Part model, mm, in its own coordinate system. Give positions to 0.01 mm unless a question says otherwise; leave off trailing zeros. Loops run counter-clockwise (first coordinate to the right, second up) from the corner with the lowest first, then second, coordinate; pieces in that order, holes last. Notation, with made-up numbers: (59, 36) -> (102, 36) arc R21 cw to (102, 43) -> close; hole circle Ø11 at (26.5, 1.25). An arc over 180 degrees is marked (long way). One line per question, with ' | ' between items.
```python
from build123d import *

# Parameters (mm, degrees)
SKETCH1_R           = 1.6
BOSS_EXTRUDE2_DEPTH = 5
BOSS_EXTRUDE3_DEPTH = 10
CHAMFER1_SIZE       = 1.5
FILLET1_R           = 10
FILLET2_R           = 1


with BuildPart() as part:
    # Sketch1 → Boss-Extrude2 (new body)
    with BuildSketch(Plane(origin=(0, 0, 0), x_dir=(0, 1, 0), z_dir=(0, 0, 1))):
        with BuildLine():
            Line((-82.0624762, -24), (82.0624762, -24))
            ThreePointArc((82.0624762, -24), (0, -85.5), (-82.0624762, -24))
        make_face()
        with Locations(Location((-20, -75, 0), (0, 0, 270))):
            Circle(SKETCH1_R, mode=Mode.SUBTRACT)
        with Locations(Location((20, -75, 0), (0, 0, 90))):
            Circle(SKETCH1_R, mode=Mode.SUBTRACT)
        with Locations(Location((-69.5, -28.2, 0), (0, 0, 270))):
            Circle(SKETCH1_R, mode=Mode.SUBTRACT)
        with Locations(Location((69.5, -28.2, 0), (0, 0, 90))):
            Circle(SKETCH1_R, mode=Mode.SUBTRACT)
    extrude(amount=BOSS_EXTRUDE2_DEPTH)

    # Sketch2 → Boss-Extrude3 (add)
    with BuildSketch(Plane.XY.offset(5)):
        with BuildLine():
            Line((60, 45), (24, 45))
            Line((24, 45), (24, 40))
            Line((24, 40), (63.442887702, 40))
            ThreePointArc((63.442887702, 40), (61.772053803, 42.534848876), (60, 45))
        make_face()
        with BuildLine():
            Line((24, -45), (24, -40))
            Line((24, -40), (63.442887702, -40))
            ThreePointArc((63.442887702, -40), (61.772053803, -42.534848876), (60, -45))
            Line((60, -45), (24, -45))
        make_face()
    extrude(amount=BOSS_EXTRUDE3_DEPTH)

    # Chamfer1
    chamfer1_edges = [part.edges().sort_by_distance(p)[0] for p in [
        (76.6, 20, 5),
        (26.6, -69.5, 5),
        (29.8, 69.5, 5),
        (73.4, -20, 5),
    ]]
    chamfer(chamfer1_edges, length=CHAMFER1_SIZE)

    # Fillet1
    fillet1_edges = [part.edges().sort_by_distance(p)[0] for p in [
        (42, -45, 5),
        (42, 45, 5),
    ]]
    fillet(fillet1_edges, radius=FILLET1_R - 0.0001)  # a hair under: the kernel refuses the full size

    # Fillet2
    fillet2_edges = [part.edges().sort_by_distance(p)[0] for p in [
        (43.721443851, 40, 5),
        (43.721443851, -40, 5),
    ]]
    fillet(fillet2_edges, radius=FILLET2_R)


solid = part.part
```
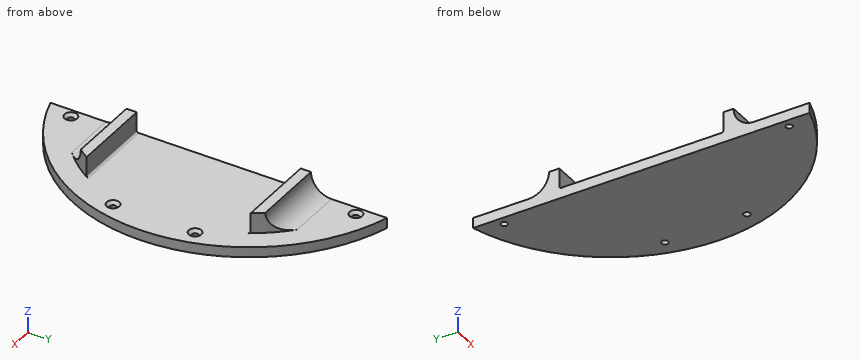
1) Pin check, flat tips, straight feed: P1, Ø4, axis at x = 42, z = 12, coming from the -Y side; P2, Ø6, axis at x = 58, z = 7, coming from the -Y side; P3, Ø4, axis at x = 75, y = -20, coming from the +Z side. Stop position of each tip, or through.
Found:
P1: y = -46.34 | P2: y = -64.81 | P3: z = 3.9
2) Saw through at C-C (x = 75). Give the cut face in (y, z), and give its area (3 significant figures).
Found:
outline: (-41.05, 0) -> (-21.6, 0) -> (-21.6, 3.5) -> (-23.1, 5) -> (-41.05, 5) -> close; (-18.4, 0) -> (18.4, 0) -> (18.4, 3.5) -> (16.9, 5) -> (-16.9, 5) -> (-18.4, 3.5) -> close; (21.6, 0) -> (41.05, 0) -> (41.05, 5) -> (23.1, 5) -> (21.6, 3.5) -> close | area: 374 mm2
3) Saw through at B-B (y = 20). Give the cut face in (x, z).
Found:
outline: (24, 0) -> (73.4, 0) -> (73.4, 3.5) -> (71.9, 5) -> (24, 5) -> close; (76.6, 0) -> (83.13, 0) -> (83.13, 5) -> (78.1, 5) -> (76.6, 3.5) -> close
4) Drill centre lines: line 1 (Y direction, x = 75, z = 1.2); line 2 (Y direction, x = 28.2, z = 0.9); line 3 (X direction, y = -47.5, z = 3.5). Where is each one in solid material? Low to high.
Found:
line 1: -41.05 to -21.6, -18.4 to 18.4, 21.6 to 41.05 | line 2: -80.72 to -71.1, -67.9 to 67.9, 71.1 to 80.72 | line 3: 24 to 71.09
5) Saw through at A-A (z = 7.5). Give the cut face in (x, y).
Found:
outline: (24, -48.39) -> (57.3, -48.39) arc R75 ccw to (63.44, -40) -> (24, -40) -> close; (24, 40) -> (63.44, 40) arc R75 ccw to (57.3, 48.39) -> (24, 48.39) -> close
